from build123d import *

# Parameters (mm, degrees)
CHAMFER1_SIZE      = 0.5
SKETCH3_R          = 3
CUT_EXTRUDE1_DEPTH = 41.155946011


with BuildPart() as part:
    # Sketch1 → Revolve2 (revolve)
    with BuildSketch(Plane(origin=(0, 0, 0), x_dir=(1, 0, 0), z_dir=(0, 1, 0)), mode=Mode.PRIVATE) as revolve2_sk:
        Polygon((0, 0), (0, 27.5), (4, 27.5), (4, 17.5), (10, 17.5), (10, 13.5), (4, 13.5), (4, 0), align=None)
    revolve(revolve2_sk.sketch.rotate(Axis((0, 0, 0), (1, 0, 0)), 180), axis=Axis((0, 0, 0), (1, 0, 0)))

    # Chamfer1
    chamfer1_edges = [part.edges().sort_by_distance(p)[0] for p in [
        (10, 0, -17.5),
    ]]
    chamfer(chamfer1_edges, length=CHAMFER1_SIZE)

    # Sketch3 → Cut-Extrude1 (cut, through all)
    with BuildSketch(Plane.ZY):
        with Locations((0, 22)):
            Circle(SKETCH3_R)
        with Locations((22, 0)):
            Circle(SKETCH3_R)
        with Locations((0, -22)):
            Circle(SKETCH3_R)
        with Locations((-22, 0)):
            Circle(SKETCH3_R)
    extrude(amount=-CUT_EXTRUDE1_DEPTH, mode=Mode.SUBTRACT)


solid = part.part
Input: part model. Units: mm. Frame: model coordinates. A direction names the side the tool comes from. Give positions to 0.01 mm unless a question says otherwise; leave off trailing zeros. Loops run counter-clockwise (first coordinate to the right, second up) from the corner with the lowest first, then second, coordinate; pieces in that order, holes last. Notation, with made-up numbers: M 65.5,-31 L 76.5,-31 A27 ccw 76.5,4 Z; hole C 2.25,72 d6. An arc over 180 degrees is marked long. Use one line per item in the form item = value.
1. Pull-direction query (Y, two-part tool) for faces 1 (the face through (2.028, 24.397, 12.69)), 2 (the face through (2, 0, -25)), 3 (the face through (4, 18, 0)), 4 (the face through (6.96, 13.18, -2.93)); classes: released by +Y, released by -Y, zero draft, split by the parting line, or undercut.
Numbers:
face_1 = split by the parting line
face_2 = undercut
face_3 = zero draft
face_4 = undercut
2. Section query C-C, the plane y = 22. Return the cut outline in (x, z).
Numbers:
outline = M 0,-16.5 L 4,-16.5 L 4,-3 L 0,-3 Z; M 0,3 L 4,3 L 4,16.5 L 0,16.5 Z
3. Section query A-A, the plane z = 0. Return the cut outline in (x, y), and give its area (3 significant figures).
Numbers:
outline = M 0,-27.5 L 4,-27.5 L 4,-25 L 0,-25 Z; M 0,-19 L 4,-19 L 4,-17.5 L 9.5,-17.5 L 10,-17 L 10,-13.5 L 4,-13.5 L 4,13.5 L 10,13.5 L 10,17 L 9.5,17.5 L 4,17.5 L 4,19 L 0,19 Z; M 0,25 L 4,25 L 4,27.5 L 0,27.5 Z
area = 220 mm²
4. Reachability of faces 5 (the face through (1.97, -24.93, -0.65)), 6 (the face through (4, 0, 0)) from +Z, -Z, +X, -X, +Y, -Y: full face, straight path, thin tool, end or side. Return the list, or none.
Numbers:
face_5 = +X, -X
face_6 = +X
5. Line query: L1, parallel to Y at x = 2.55, z = 0; L2, parallel to Y at x = 7, z = 0.5; L3, parallel to Z at x = 3.5, y = 2. Output: solid intervals per line, ascending.
Numbers:
L1 = -27.5 to -25, -19 to 19, 25 to 27.5
L2 = -17.49 to -13.49, 13.49 to 17.49
L3 = -27.43 to -24.24, -19.76 to 19.76, 24.24 to 27.43
6. Section query D-D, the plane x = 2.75. Return the cut outline in (y, z), and give its area (3 significant figures).
Numbers:
outline = C 0,0 d55; hole C -22,0 d6; hole C 0,-22 d6; hole C 0,22 d6; hole C 22,0 d6
area = 2,260 mm²
7. First-contact query: pin 1 (21.5 mm diameter, centred on y = 3, z = 0.5, fed in from +X); pin 2 (1.5 mm diameter, centred on x = 6, z = -12.5, fed in from -Y); pin 3 (6 mm diameter, centred on y = 3.5, z = -2, fed in from +X); pin 4 (1.5 mm diameter, centred on x = 3.5, y = 19, fed in from +Z). Flat tips, straight axial feed; report the tip coordinate or a pass-through.
Numbers:
pin_1 = 10
pin_2 = -12.97
pin_3 = 4
pin_4 = 20.57
